Geometry: final body of the model. Coordinates: model frame, mm. Face numbers are marked on the shaded views. A direction names the side the tool comes from. Give positions to 0.01 mm unless a question says otherwise; leave off trailing zeros. Write each loop counter-clockwise with the first axis right and the second up, starting at its lowest first coordinate (ties: lowest second). Pieces come first, ordered by that corner, then holes.
Q1. Cut plane D-D on z = 18.25. Return the cut outline in (x, y), plus the area to 3 significant figures.
Q2. Line query: L1, parallel to Y at x = 0, z = 14.75; L2, parallel to X at y = 4.5, z = 23.25; L3, parallel to Y at x = -34, z = 26.75. Output: solid intervals per line, ascending.
Q3. Pin query (flat end, axial travel): pin 1 (3 mm diameter, centred on x = -34.66, z = 24.56, fed in from -Y); pin 2 (0.8 mm diameter, centred on x = -45, z = 5, fed in from +Y); pin 3 (3 mm diameter, centred on x = -45, z = 5, fed in from +Y); pin 4 (1.5 mm diameter, centred on x = -23, y = -3.5, fed in from -Z). Return the tip coordinate at first contact, or that it passes through.
Q4. Draft query along X for the marked faces 1 and 2. Return one class per face: pulls with the +X half, pulls with the -X half, needs draft (parallel to the pull), parting line crosses it, or undercut.
Q5. Reachability of the marked faces 3, 4 and 5 from +Z, -Z, +X, -X, +Y, -Y: full face, straight path, thin tool, end or side. Return the list, or none.
Q6. Cut plane B-B on z = 5. Return the cut outline in (x, y).
Q7. Cut plane C-C on x = -45. Return the cut outline in (y, z), plus the area to 4 significant figures.
Q8. Cut plane A-A on x = 0. Return the cut outline in (y, z), plus the area to 3 significant figures.
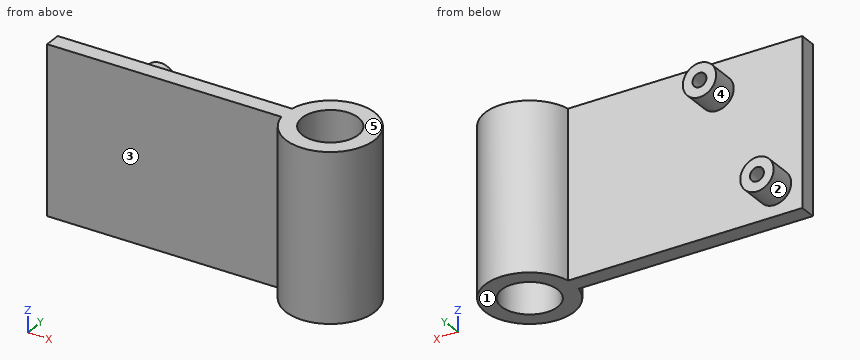
```python
from build123d import *

# Parameters (mm, degrees)
SKETCH1_R           = 5.05
BOSS_EXTRUDE1_DEPTH = 30
SKETCH2_R           = 3
SKETCH2_R_2         = 1.25
BOSS_EXTRUDE2_DEPTH = 5


with BuildPart() as part:
    # Sketch1 → Boss-Extrude1 (new body)
    with BuildSketch(Plane.XY):
        with BuildLine():
            Line((-7.858116823, 1.5), (-50, 1.5))
            Line((-50, 1.5), (-50, -1.5))
            Line((-50, -1.5), (-7.858116823, -1.5))
            ThreePointArc((-7.858116823, -1.5), (8, 0), (-7.858116823, 1.5))
        make_face()
        Circle(SKETCH1_R, mode=Mode.SUBTRACT)
    extrude(amount=BOSS_EXTRUDE1_DEPTH)

    # Sketch2 → Boss-Extrude2 (add)
    # profile 1 of 2: a face of its own
    with BuildSketch(Plane(origin=(0, 1.5, 0), x_dir=(1, 0, 0), z_dir=(0, 1, 0))):
        with Locations(Location((-45, -5, 0), (0, 0, 90))):
            Circle(SKETCH2_R)
        with Locations(Location((-45, -5, 0), (0, 0, 270))):
            Circle(SKETCH2_R_2, mode=Mode.SUBTRACT)
    # profile 2 of 2: a face of its own
    with BuildSketch(Plane(origin=(0, 1.5, 0), x_dir=(1, 0, 0), z_dir=(0, 1, 0))):
        with Locations(Location((-34.6622, -24.558, 0), (0, 0, 90))):
            Circle(SKETCH2_R)
        with Locations(Location((-34.6622, -24.558, 0), (0, 0, 270))):
            Circle(SKETCH2_R_2, mode=Mode.SUBTRACT)
    extrude(amount=BOSS_EXTRUDE2_DEPTH)


solid = part.part
```
Data:
1. outline: (-50, -1.5) - (-7.86, -1.5) arc R8 ccw (long way) to (-7.86, 1.5) - (-50, 1.5) - close; hole circle Ø10.1 at (0, 0)
1. area: 247 mm2
2. L1: y = -8 to -5.05, 5.05 to 8
2. L2: x = -37.36 to -31.96, -6.61 to -2.29, 2.29 to 6.61
2. L3: y = -1.5 to 6.5
3. pin 1: stops at y = -1.5
3. pin 2: stops at y = 1.5
3. pin 3: stops at y = 6.5
3. pin 4: passes through
4. face 1: needs draft
4. face 2: undercut
5. face 3: +Z, -Z, -X, -Y
5. face 4: +Y
5. face 5: +Z, +X, -X, +Y, -Y
6. outline: (-50, -1.5) - (-7.86, -1.5) arc R8 ccw (long way) to (-7.86, 1.5) - (-42, 1.5) - (-42, 6.5) - (-43.75, 6.5) - (-43.75, 1.5) - (-46.25, 1.5) - (-46.25, 6.5) - (-48, 6.5) - (-48, 1.5) - (-50, 1.5) - close; hole circle Ø10.1 at (0, 0)
7. outline: (-1.5, 0) - (1.5, 0) - (1.5, 2) - (6.5, 2) - (6.5, 3.75) - (1.5, 3.75) - (1.5, 6.25) - (6.5, 6.25) - (6.5, 8) - (1.5, 8) - (1.5, 30) - (-1.5, 30) - close
7. area: 107.5 mm2
8. outline: (-8, 0) - (-5.05, 0) - (-5.05, 30) - (-8, 30) - close; (5.05, 0) - (8, 0) - (8, 30) - (5.05, 30) - close
8. area: 177 mm2
